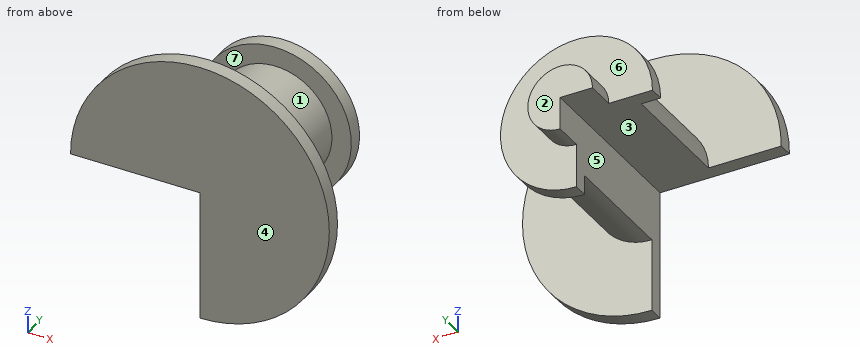
```python
from build123d import *

# Parameters (mm, degrees)
REVOLVE1_ANGLE = 270


with BuildPart() as part:
    # Sketch1 → Revolve1 (revolve)
    with BuildSketch(Plane.XY):
        Polygon((0, 0), (-80, 0), (-80, 9), (-35, 9), (-35, 83), (-47, 83), (-47, 92), (-20, 92), (-20, 110), (0, 110), align=None)
    revolve(axis=Axis((0, 0, 0), (0, 1, 0)), revolution_arc=REVOLVE1_ANGLE)


solid = part.part
```
The model under review builds one solid part; all positions refer to its coordinate system, in mm. Face numbers are marked on the shaded views. A direction names the side the tool comes from. Round coordinates to 2 decimals unless told otherwise and drop trailing zeros. Write each loop counter-clockwise with the first axis right and the second up, starting at its lowest first coordinate (ties: lowest second). Pieces come first, ordered by that corner, then holes. Notation, with made-up numbers: (-4, -30.75) - (15, -30.75) arc R27 ccw to (15, 6.25) - close; hole circle Ø3 at (70, 18). An arc over 180 degrees is marked (long way). Answer as CSV lines item,"result". Start each with the question number.
(1) Draft analysis for pull direction Y (two halves, no side actions). For the marked faces 4, 5, 6 and 7, state which applies: pulls with the +Y half, pulls with the -Y half, needs draft (parallel to the pull), parting line crosses it, or undercut.
(2) For pin 1 Ø5 at (x, y) = (2, 62.5) entering from +Z; pin 2 Ø4 at (x, y) = (11.5, 45.5) entering from +Z; pin 3 Ø10 at (x, z) = (23, 48.5) entering from +Y, all flat-tipped, find the tip position at first contact; note any pin that passes through.
(3) To check wall thickness, follow line 1 (Y direction, x = -40, z = 6.5); line 2 (Y direction, x = -73, z = 6.5); line 3 (Z direction, x = -24, y = 84). State the ranges of each line that lie inside material, in increasing order.
(4) We need section B-B on z = -28.5. State the section outline as (x, y) points, plus the area to 3 significant figures.
(5) For the marked faces 1, 2 and 3, list the 3-axis set-ups (+Z, -Z, +X, -X, +Y, -Y) from which the entire face can be reached by the end or side of a thin tool; tool diameter is ignored.
(6) We need section A-A on x = 44. State the section outline as (y, z) points.
(7) We need section D-D on x = -6.5. State the section outline as (y, z) points, plus the area to 3 significant figures.
(8) We need section C-C on y = 42.5. State the section outline as (x, z) points.
Worked answers:
1,face 4,"pulls with the -Y half"
1,face 5,"needs draft"
1,face 6,"pulls with the +Y half"
1,face 7,"undercut"
2,pin 1,"z = 35"
2,pin 2,"z = 33.69"
2,pin 3,"y = 9"
3,line 1,"0 to 9, 83 to 92"
3,line 2,"0 to 9"
3,line 3,"0 to 40.41"
4,outline,"(0, 0) - (74.75, 0) - (74.75, 9) - (20.32, 9) - (20.32, 83) - (37.37, 83) - (37.37, 92) - (0, 92) - close"
4,area,"2,510 mm²"
5,face 1,"none"
5,face 2,"+Z, -Z, +X, -X, +Y"
5,face 3,"-Z, -X, +Y, -Y"
6,outline,"(0, -66.81) - (9, -66.81) - (9, 66.81) - (0, 66.81) - close; (83, -16.52) - (92, -16.52) - (92, 16.52) - (83, 16.52) - close"
7,outline,"(0, 0) - (110, 0) - (110, 18.91) - (92, 18.91) - (92, 46.55) - (83, 46.55) - (83, 34.39) - (9, 34.39) - (9, 79.74) - (0, 79.74) - close"
7,area,"4,020 mm²"
8,outline,"(-35, 0) - (0, 0) - (0, -35) arc R35 ccw (long way) to start"
